The listing builds one solid part. Answer for the finished solid, in the listing's coordinates (mm). Face numbers are marked on the shaded views. A direction names the side the tool comes from. Coordinates: 2 decimals unless noted, no trailing zeros. Write each loop counter-clockwise with the first axis right and the second up, starting at its lowest first coordinate (ties: lowest second). Pieces come first, ordered by that corner, then holes. Notation, with made-up numbers: M 1,50.25 L 22,50.25 A28 cw 22,72.25 Z; hole C 62,-24.75 d5. An arc over 180 degrees is marked long. Answer as a JSON object with one key per item and string values. Group by question number.
from build123d import *

# Parameters (mm, degrees)
F0_W     = 27.2240719226
F0_H     = 2
F1_DEPTH = 3
F2_DEPTH = 10
F3_R     = 1.5
F4_R     = 1
F5_R     = 3
F6_R     = 5


with BuildPart() as f1:
    # F0 (on Top) → F1 (new body)
    with BuildSketch(Plane.XY):
        Polygon((-7.7136544558, 22.5634722376), (-7.7136544558, 47.5634722376), (-47.7136544558, 45.1496791341), (-47.7136544558, 24.977265341), align=None)
        with Locations((-29.1016184945, 32.6534722376)):
            Rectangle(F0_W, F0_H, mode=Mode.SUBTRACT)
        with Locations((-29.1016184945, 37.4734722376)):
            Rectangle(F0_W, F0_H, mode=Mode.SUBTRACT)
    extrude(amount=F1_DEPTH)

    # F0 (on Top) → F2 (join)
    with BuildSketch(Plane.XY):
        with Locations((-29.1016184945, 32.6534722376)):
            Rectangle(F0_W, F0_H)
        with Locations((-29.1016184945, 37.4734722376)):
            Rectangle(F0_W, F0_H)
    extrude(amount=F2_DEPTH)

    # F3
    f3_edges = [f1.edges().sort_by_distance(p)[0] for p in [
        (-42.713654, 36.473472, 6.5),
        (-42.713654, 33.653472, 6.5),
        (-15.489583, 36.473472, 6.5),
        (-15.489583, 33.653472, 6.5),
    ]]
    fillet(f3_edges, radius=F3_R)

    # F4
    f4_edges = [f1.edges().sort_by_distance(p)[0] for p in [
        (-29.101618, 36.473472, 10),
        (-29.101618, 33.653472, 10),
        (-42.713654, 31.903472, 10),
        (-42.274315, 33.214132, 10),
        (-15.489583, 31.903472, 10),
        (-15.928922, 33.214132, 10),
        (-15.928922, 36.912812, 10),
        (-42.274315, 36.912812, 10),
        (-15.489583, 38.223472, 10),
        (-42.713654, 38.223472, 10),
    ]]
    fillet(f4_edges, radius=F4_R)

    # F5
    f5_edges = [f1.edges().sort_by_distance(p)[0] for p in [
        (-7.713654, 22.563472, 1.5),
        (-7.713654, 47.563472, 1.5),
    ]]
    fillet(f5_edges, radius=F5_R)

    # F6
    f6_edges = [f1.edges().sort_by_distance(p)[0] for p in [
        (-47.713654, 45.149679, 1.5),
        (-47.713654, 24.977265, 1.5),
    ]]
    fillet(f6_edges, radius=F6_R)


solid = f1.part
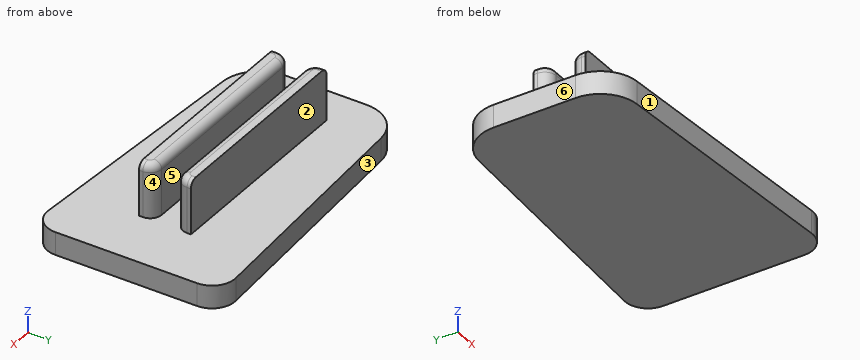
Item 1: A cutting plane is placed at B-B, the plane y = 35.75. Write down the section's boundary in (x, z), and give its area (3 significant figures).
Item 2: A tool of negligible diameter and unlimited length cuts with its end or side. For the marked faces 1 and 2, from which of +Z, -Z, +X, -X, +Y, -Y can it reach the whole face along a straight path? Write none if from no direction.
Item 3: Flat-ended cylindrical pins translate along their axes: pin 1 Ø1.5 at (y, z) = (26, 4.5) entering from +X; pin 2 Ø12 at (x, y) = (-29, 25.5) entering from +Z; pin 3 Ø2 at (x, z) = (-38, 4.5) entering from -Y; pin 4 Ø3.5 at (x, z) = (-27, 8) entering from +Y. Find the tip coordinate at first contact, or state that the pin passes through.
Item 4: A cutting plane is placed at D-D, the plane y = 42.5. Write down the section's boundary in (x, z), and give its area (3 significant figures).
Item 5: A cutting plane is placed at A-A, the plane z = 7.5. Write down the section's boundary in (x, y), and give its area (3 significant figures).
Item 6: For a pull along Y with two mould halves and no side action, classify the marked faces 3, 4, 5 and 6 as +Y half, -Y half, draft (parallel to the pull), parting line (faces both ways), or undercut.
Item 7: Consider L1, parallel to Y at x = -20, z = 6.25; L2, parallel to X at y = 32, z = 8.5; L3, parallel to Z at x = -37, y = 45.5. Determine where each line is inside the solid, lowest interval first. Write a range as from..to.
Item 8: A cutting plane is placed at C-C, the plane x = -34. Write down the section's boundary in (y, z).
Answer:
{
 "1": {"outline": "M -47.71,0 L -7.71,0 L -7.71,3 L -47.71,3 Z", "area": "120 mm2"},
 "2": {"face 1": "+Z, -Z, -X, -Y", "face 2": "+Z, +X, -X, +Y"},
 "3": {"pin 1": "through", "pin 2": "z = 3", "pin 3": "y = 31.65", "pin 4": "y = 38.47"},
 "4": {"outline": "M -47.27,0 L -7.71,0 L -7.71,3 L -47.27,3 Z", "area": "119 mm2"},
 "5": {"outline": "M -42.71,31.65 L -15.49,31.65 L -15.49,32.15 A1.5 ccw -16.99,33.65 L -41.21,33.65 A1.5 ccw -42.71,32.15 Z; M -42.71,37.97 A1.5 ccw -41.21,36.47 L -16.99,36.47 A1.5 ccw -15.49,37.97 L -15.49,38.47 L -42.71,38.47 Z", "area": "107 mm2"},
 "6": {"face 3": "+Y half", "face 4": "undercut", "face 5": "undercut", "face 6": "draft"},
 "7": {"L1": "31.65..33.65, 36.47..38.47", "L2": "-42.71..-15.49", "L3": "0..3"},
 "8": {"outline": "M 24.15,0 L 45.98,0 L 45.98,3 L 38.47,3 L 38.47,10 L 37.47,10 A1 ccw 36.47,9 L 36.47,3 L 33.65,3 L 33.65,9 A1 ccw 32.65,10 L 31.65,10 L 31.65,3 L 24.15,3 Z"}
}
